```python
from build123d import *

# Parameters (mm, degrees)
SKETCH1_R             = 0.3
BOSS_EXTRUDE1_DEPTH   = 3.8
BOSS_EXTRUDE1_2_DEPTH = 3.8
BOSS_EXTRUDE1_3_DEPTH = 3.8
SKETCH2_W             = 7.5
SKETCH2_H             = 14.1
BOSS_EXTRUDE2_DEPTH   = 8.1
SKETCH3_W             = 3
SKETCH3_H             = 3
BOSS_EXTRUDE3_DEPTH   = 6


with BuildPart() as part:
    # Sketch1 → Boss-Extrude1 (new body)
    with BuildSketch(Plane(origin=(0, 0, 0), x_dir=(1, 0, 0), z_dir=(0, 1, 0))):
        Circle(SKETCH1_R)
    extrude(amount=-BOSS_EXTRUDE1_DEPTH)



with BuildPart() as body_2:
    # Sketch1 → Boss-Extrude1 2 (new body)
    with BuildSketch(Plane(origin=(0, 0, 0), x_dir=(1, 0, 0), z_dir=(0, 1, 0))):
        with Locations((0, -2.54)):
            Circle(SKETCH1_R)
    extrude(amount=-BOSS_EXTRUDE1_2_DEPTH)


with BuildPart() as body_3:
    # Sketch1 → Boss-Extrude1 3 (new body)
    with BuildSketch(Plane(origin=(0, 0, 0), x_dir=(1, 0, 0), z_dir=(0, 1, 0))):
        with Locations((0, 2.54)):
            Circle(SKETCH1_R)
    extrude(amount=-BOSS_EXTRUDE1_3_DEPTH)


with BuildPart() as part_1:
    add(part.part)

    add(body_2.part)  # Boss-Extrude2 merges body 2

    add(body_3.part)  # Boss-Extrude2 merges body 3
    # Sketch2 → Boss-Extrude2 (add)
    with BuildSketch(Plane(origin=(0, 0, 0), x_dir=(1, 0, 0), z_dir=(0, 1, 0))):
        Rectangle(SKETCH2_W, SKETCH2_H)
    extrude(amount=BOSS_EXTRUDE2_DEPTH)

    # Sketch3 → Boss-Extrude3 (add)
    with BuildSketch(Plane.ZY.offset(3.75)):
        with Locations((-3, 5.8)):
            Rectangle(SKETCH3_W, SKETCH3_H)
    extrude(amount=BOSS_EXTRUDE3_DEPTH)


solid = part_1.part
```
Verification items for the finished model (mm, model axes). A direction names the side the tool comes from. Coordinates: 2 decimals unless noted, no trailing zeros. Write each loop counter-clockwise with the first axis right and the second up, starting at its lowest first coordinate (ties: lowest second). Pieces come first, ordered by that corner, then holes. Notation, with made-up numbers: (67, -8) - (111, -8) arc R10 ccw to (111, 10) - close; hole circle Ø4 at (11.5, -18.5). An arc over 180 degrees is marked (long way). Write item = value, one per line.
Q1. Access from +Z, -Z, +X, -X, +Y, -Y to the whole of each face (thin tool, end or side, straight path). Record for faces 1 (the face through (-7, 7.3, -3)), 2 (the face through (-7, 6, -1.5)), 3 (the face through (-7, 4.3, -3)), 4 (the face through (-7, 6, -4.5)).
Answer:
face_1 = +Z, -Z, -X, +Y
face_2 = +Z, -X, +Y, -Y
face_3 = +Z, -Z, -X, -Y
face_4 = -Z, -X, +Y, -Y
Q2. Cross-section at C-C (y = 5.5). Enter the section's corners in (x, z), plus the area to 3 significant figures.
Answer:
outline = (-9.75, -4.5) - (-3.75, -4.5) - (-3.75, -7.05) - (3.75, -7.05) - (3.75, 7.05) - (-3.75, 7.05) - (-3.75, -1.5) - (-9.75, -1.5) - close
area = 124 mm²
Q3. Cross-section at D-D (x = 0). Enter the section's corners in (y, z).
Answer:
outline = (-3.8, -2.84) - (0, -2.84) - (0, -7.05) - (8.1, -7.05) - (8.1, 7.05) - (0, 7.05) - (0, 2.84) - (-3.8, 2.84) - (-3.8, 2.24) - (0, 2.24) - (0, 0.3) - (-3.8, 0.3) - (-3.8, -0.3) - (0, -0.3) - (0, -2.24) - (-3.8, -2.24) - close
Q4. Go/stop test with flat-tipped pins: pin 1 Ø1.5 at (x, z) = (-6.5, -3.5) entering from -Y; pin 2 Ø3.5 at (x, y) = (-6, 5.5) entering from -Z; pin 3 Ø1 at (y, z) = (1.5, 4) entering from -X. Record where each tip stops, or that it passes through.
Answer:
pin_1 = 4.3
pin_2 = -4.5
pin_3 = -3.75
Q5. Cross-section at A-A (z = -3.25). Enter the section's corners in (x, y).
Answer:
outline = (-9.75, 4.3) - (-3.75, 4.3) - (-3.75, 0) - (3.75, 0) - (3.75, 8.1) - (-3.75, 8.1) - (-3.75, 7.3) - (-9.75, 7.3) - close
Q6. Material ranges on L1, parallel to Y at x = 3.25, z = -3; L2, parallel to X at y = 5.25, z = 6; L3, parallel to Y at x = -5.5, z = -4.25, recorded low to high. Write a range as from..to.
Answer:
L1 = 0..8.1
L2 = -3.75..3.75
L3 = 4.3..7.3
Q7. Cross-section at B-B (y = -0.5). Enter the section's corners in (x, z).
Answer:
outline = circle Ø0.6 at (0, -2.54); circle Ø0.6 at (0, 0); circle Ø0.6 at (0, 2.54)
